from build123d import *

# Parameters (mm, degrees)
SKETCH1_R               = 12
BOSS_EXTRUDE1_DEPTH     = 80
SHELL1_T                = -3.175
SKETCH3_R               = 1.5
CUT_EXTRUDE1_DEPTH      = 82.780193201
CUT_EXTRUDE1_DEPTH_BACK = 82.780193201


with BuildPart() as part:
    # Sketch1 → Boss-Extrude1 (new, symmetric)
    with BuildSketch(Plane.XY):
        Circle(SKETCH1_R)
    extrude(amount=BOSS_EXTRUDE1_DEPTH, both=True)

    # Shell1
    shell1_openings = [part.faces().sort_by_distance(p)[0] for p in [
        (0, 0, 80),
        (0, 0, -80),
    ]]
    offset(amount=SHELL1_T, openings=shell1_openings, kind=Kind.INTERSECTION)

    # Sketch3 → Cut-Extrude1 (cut, two sides)
    with BuildSketch(Plane(origin=(0, 0, 0), x_dir=(1, 0, 0), z_dir=(0, 1, 0))) as cut_extrude1_sk:
        with Locations(Location((0, 28, 0), (0, 0, 270))):
            Circle(SKETCH3_R)
        with Locations(Location((0, -28, 0), (0, 0, 270))):
            Circle(SKETCH3_R)
        with Locations(Location((0, -43, 0), (0, 0, 270))):
            Circle(SKETCH3_R)
        with Locations(Location((0, 43, 0), (0, 0, 270))):
            Circle(SKETCH3_R)
    extrude(amount=CUT_EXTRUDE1_DEPTH, mode=Mode.SUBTRACT)
    extrude(cut_extrude1_sk.sketch, amount=-CUT_EXTRUDE1_DEPTH_BACK, mode=Mode.SUBTRACT)


solid = part.part
Design review of the part built by this model. Coordinates are the model's own, in mm. Give positions to 0.01 mm unless a question says otherwise; leave off trailing zeros. Loops run counter-clockwise (first coordinate to the right, second up) from the corner with the lowest first, then second, coordinate; pieces in that order, holes last. Notation, with made-up numbers: M 74.25,2.25 L 103.25,2.25 A27 ccw 103.25,29.25 Z; hole C 13.25,77.25 d7. An arc over 180 degrees is marked long. One line per question, with ' | ' between items. Start each with the question number.
1. Add section D-D (z = 9). Write out the cut boundary in (x, y) (3 decimals), plus the area to 3 significant figures.
2. Add section C-C (x = 0). Give the number of separate pieces and of enclosed holes in the cut face, plus the area to 3 significant figures.
3. Add section B-B (y = 1.75). Write out the cut boundary in (x, z).
4. Insertion check: P1, Ø1.8, axis at x = 0, z = 28, coming from the -Y side; P2, Ø1, axis at y = 9, z = 53, coming from the -X side; P3, Ø3, axis at x = -6, z = 53, coming from the -Y side; P4, Ø6, axis at y = -4, z = -54, coming from the -X side. Each pin has a flat end and moves straight along its axis. Give the tip position at first contact, or say it passes through.
5. Add section A-A (z = 28). Write out the cut boundary in (x, y) (3 decimals), plus the area to 3 significant figures.
6. To check wall thickness, follow L1, parallel to Z at x = 0, y = 9.55; L2, parallel to Y at x = -0.5, z = -59.5; L3, parallel to Y at x = 5.75, z = 62. State the ranges of each line that lie inside material, in increasing order.
7. The part is to be moulded in two halves that separate along X. For faces 1 (the face through (-11.99, 0.53, 1.12)), 2 (the face through (0, 9, 80)), 3 (the face through (0.07, 10.33, 41.5)), say which applies: released by +X, released by -X, zero draft, split by the parting line, or undercut.
Worked out:
1) outline: C 0,0 d24; hole C 0,0 d17.65 | area: 208 mm²
2) separate pieces: 10 | enclosed holes: 0 | area: 940 mm²
3) outline: M -11.87,-80 L -8.65,-80 L -8.65,80 L -11.87,80 Z; M 8.65,-80 L 11.87,-80 L 11.87,80 L 8.65,80 Z
4) P1: passes through | P2: stops at x = -8.47 | P3: stops at y = -11.12 | P4: stops at x = -11.96
5) outline: M -1.5,-11.906 L -1.5,-8.697 A8.825 cw -1.5,8.697 L -1.5,11.906 A12 ccw Z; M 1.5,-11.906 A12 ccw 1.5,11.906 L 1.5,8.697 A8.825 cw 1.5,-8.697 Z | area: 189 mm²
6) L1: z = -80 to -44.5, -41.5 to -29.5, -26.5 to 26.5, 29.5 to 41.5, 44.5 to 80 | L2: y = -11.99 to -8.81, 8.81 to 11.99 | L3: y = -10.53 to -6.69, 6.69 to 10.53
7) face 1: split by the parting line | face 2: zero draft | face 3: undercut
